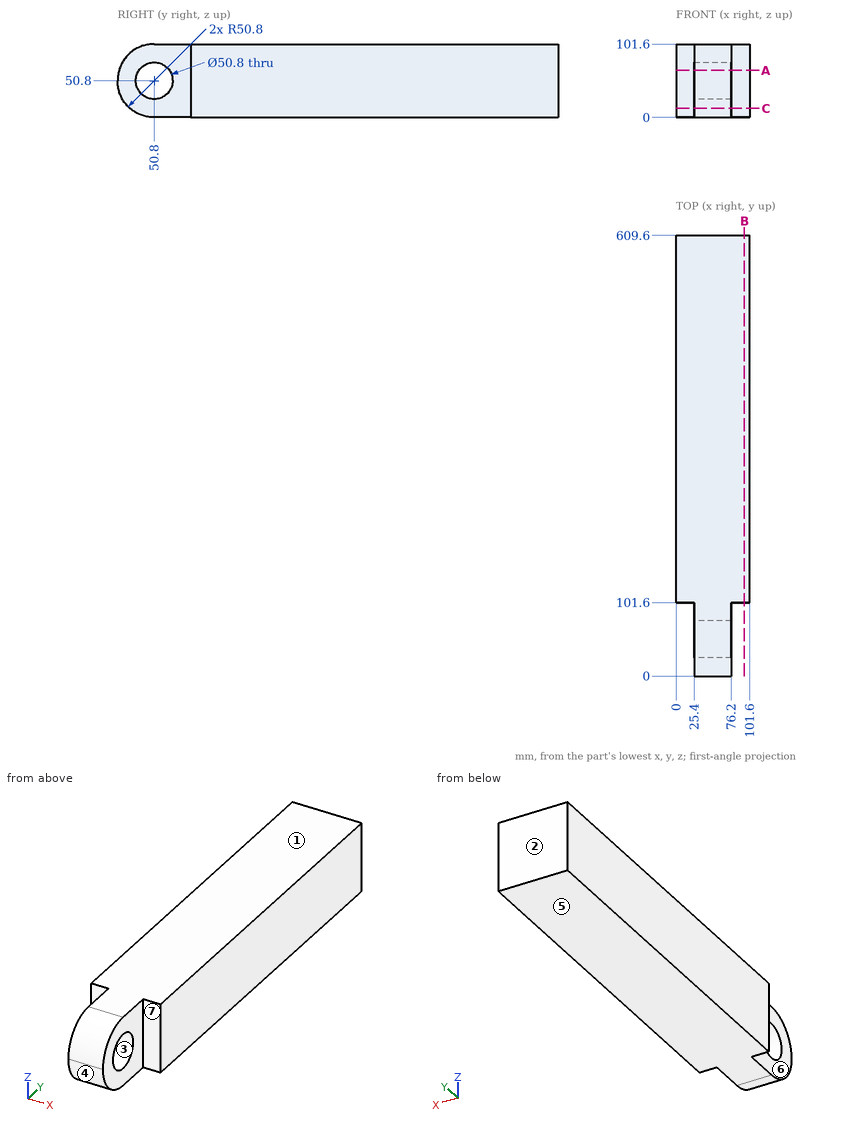
Job drawing, mm, ordinate dimensions from the low corner. One solid piece. A direction names the side the tool comes from. Round coordinates to 2 decimals unless told otherwise and drop trailing zeros. Loops run counter-clockwise (first coordinate to the right, second up) from the corner with the lowest first, then second, coordinate; pieces in that order, holes last.
(1) Which spindle directions (+Z, -Z, +X, -X, +Y, -Y) get a long thin tool onto all of the face, cutting with end or side? Do the marked faces 5, 6 and 7. Say none if no direction does.
(2) Cut at B-B (x = 94.5). Give the cut face in (y, z).
(3) Two-plate mould, pull along Z, no slides. Class the marked faces 1, 2, 3 and 4: +Z half, -Z half, draft (parallel to the pull), parting line (faces both ways), or undercut.
(4) Cut at A-A (z = 65). Give the cut face in (x, y) (3 decimals).
(5) Drop flat-ended pins along their axis: pin 1 (6 mm diameter, centred on x = 59.5, z = 14.5, fed in from -Y); pin 2 (5 mm diameter, centred on x = 89, z = 79, fed in from -Y). Give the stop position or say it passes through.
(6) Wall check: line 1 along Y through (x, z) = (42, 50.8); line 2 along Z through (x, y) = (53, 50); line 3 along Y through (x, z) = (94.5, 35). Give the ranges that are in metal, low to high.
(7) Cut at C-C (z = 12.5). Give the cut face in (x, y), plus the area to 3 significant figures.
Findings below:
1. face 5: -Z, +X, -X, +Y, -Y
1. face 6: +Z, -Z, -X, -Y
1. face 7: +Z, -Z, +X, -Y
2. outline: (101.6, 0) - (609.6, 0) - (609.6, 101.6) - (101.6, 101.6) - close
3. face 1: +Z half
3. face 2: draft
3. face 3: undercut
3. face 4: -Z half
4. outline: (0, 101.6) - (25.4, 101.6) - (25.4, 71.86) - (76.2, 71.86) - (76.2, 101.6) - (101.6, 101.6) - (101.6, 609.6) - (0, 609.6) - close; (25.4, 2.025) - (76.2, 2.025) - (76.2, 29.74) - (25.4, 29.74) - close
5. pin 1: stops at y = 12.44
5. pin 2: stops at y = 101.6
6. line 1: y = 0 to 25.4, 76.2 to 609.6
6. line 2: z = 0.01 to 25.41, 76.19 to 101.59
6. line 3: y = 101.6 to 609.6
7. outline: (0, 101.6) - (25.4, 101.6) - (25.4, 17.43) - (76.2, 17.43) - (76.2, 101.6) - (101.6, 101.6) - (101.6, 609.6) - (0, 609.6) - close
7. area: 55,900 mm2
